```python
from build123d import *

# Parameters (mm, degrees)
SKETCH_1_W          = 20
SKETCH_1_H          = 20
EXTRUDE_1_DEPTH     = 100
SKETCH_2_R          = 2.1
CUT_EXTRUDE_1_DEPTH = 103.46950766
SKETCH_4_W          = 18
SKETCH_4_H          = 18
CUT_EXTRUDE_2_DEPTH = 101.995049384


with BuildPart() as part:
    # 草图1 → 凸台-拉伸1 (new body)
    with BuildSketch(Plane.XY):
        Rectangle(SKETCH_1_W, SKETCH_1_H)
    extrude(amount=EXTRUDE_1_DEPTH)

    # 草图2 → 切除-拉伸1 (cut, through all)
    with BuildSketch(Plane(origin=(10, 0, 0), x_dir=(0, 0, -1), z_dir=(1, 0, 0))):
        with Locations((-10, 0)):
            Circle(SKETCH_2_R)
        with Locations((-30, 0)):
            Circle(SKETCH_2_R)
        with Locations(Location((-90, 0, 0), (0, 0, 180))):
            Circle(SKETCH_2_R)
        with Locations(Location((-70, 0, 0), (0, 0, 180))):
            Circle(SKETCH_2_R)
    extrude(amount=-CUT_EXTRUDE_1_DEPTH, mode=Mode.SUBTRACT)

    # 草图4 → 切除-拉伸2 (cut, through all)
    with BuildSketch(Plane(origin=(0, 0, 0), x_dir=(-1, 0, 0), z_dir=(0, 0, -1))):
        Rectangle(SKETCH_4_W, SKETCH_4_H)
    extrude(amount=-CUT_EXTRUDE_2_DEPTH, mode=Mode.SUBTRACT)


solid = part.part
```
Geometry check sheet. Reference: the model listing, model coordinates, mm. A direction names the side the tool comes from. Give positions to 0.01 mm unless a question says otherwise; leave off trailing zeros. Write each loop counter-clockwise with the first axis right and the second up, starting at its lowest first coordinate (ties: lowest second). Pieces come first, ordered by that corner, then holes.
1) Access from +Z, -Z, +X, -X, +Y, -Y to the whole of each face (thin tool, end or side, straight path). Record for faces 4 (the cylindrical face through (-9.493, -1.278, 31.666)), 5 (the flat face through (-9, 0, 49)).
2) Section check A-A, the plane y = 5.5. Record the boundary of the cut face in (x, z).
3) Section check D-D, the plane z = 17.5. Record the boundary of the cut face in (x, y), and give its area (3 significant figures).
4) Material ranges on L1, parallel to Y at x = 9.65, z = 10; L2, parallel to X at y = -7, z = 87.5, recorded low to high.
5) Release check for a two-part mould opening along X. For faces 1 (the flat face through (10, 0, 49)), 2 (the cylindrical face through (9.507, -1.278, 31.666)), 3 (the flat face through (0, -9, 49)) record: pulls with the +X half, pulls with the -X half, needs draft (parallel to the pull), parting line crosses it, or undercut.
6) Section check C-C, the plane z = 30. Record the boundary of the cut face in (x, y), and give its area (3 significant figures).
Computed:
1. face 4: +X, -X
1. face 5: +Z, -Z
2. outline: (-10, 0) - (-9, 0) - (-9, 100) - (-10, 100) - close; (9, 0) - (10, 0) - (10, 100) - (9, 100) - close
3. outline: (-10, -10) - (10, -10) - (10, 10) - (-10, 10) - close; hole (-9, -9) - (9, -9) - (9, 9) - (-9, 9) - close
3. area: 76.0 mm2
4. L1: y = -10 to -2.1, 2.1 to 10
4. L2: x = -10 to -9, 9 to 10
5. face 1: pulls with the +X half
5. face 2: needs draft
5. face 3: undercut
6. outline: (-10, -10) - (10, -10) - (10, -2.1) - (9, -2.1) - (9, -9) - (-9, -9) - (-9, -2.1) - (-10, -2.1) - close; (-10, 2.1) - (-9, 2.1) - (-9, 9) - (9, 9) - (9, 2.1) - (10, 2.1) - (10, 10) - (-10, 10) - close
6. area: 67.6 mm2
